Can you work these out from the model? Positions are in its coordinate system, mm. A direction names the side the tool comes from. Give positions to 0.01 mm unless a question says otherwise; leave off trailing zeros. Order: outer loops, then holes, each group sorted by start corner. A loop starts at its lowest first (then second) coordinate and runs counter-clockwise, first axis right, second up. Notation, with made-up numbers: (65.5, -12) -> (117.5, -12) arc R33 cw to (117.5, 20) -> close; hole circle Ø11 at (-12.75, -12). An arc over 180 degrees is marked (long way). Answer as CSV lines item,"result".
```python
from build123d import *

# Parameters (mm, degrees)
BOSS_EXTRUDE1_DEPTH = 5
SCALE2_SCALE        = 1.55
CUT_EXTRUDE1_DEPTH  = 12.4
BOSS_EXTRUDE3_DEPTH = 7.75
SKETCH9_W           = 20.224703408
SKETCH9_H           = 7.75
BOSS_EXTRUDE4_DEPTH = 29.5
CUT_EXTRUDE2_DEPTH  = 12.4
CHAMFER1_START      = -43
CHAMFER1_OUTLINE_W  = 8
CHAMFER1_OUTLINE_H  = 7.75
CHAMFER1_DEPTH      = 3.964353462
CHAMFER2_START      = 28.071920063
CHAMFER2_OUTLINE_W  = 8
CHAMFER2_OUTLINE_H  = 11
CHAMFER2_DEPTH      = 3.928079937
SKETCH11_R          = 0.8
CUT_EXTRUDE3_DEPTH  = 12.4
SKETCH12_R          = 0.8
CUT_EXTRUDE4_DEPTH  = 12.4
BOSS_EXTRUDE5_DEPTH = 14
SKETCH18_W          = 12
SKETCH18_H          = 3
BOSS_EXTRUDE6_DEPTH = 14
SKETCH19_R          = 2.4
BOSS_EXTRUDE7_DEPTH = 2.5
SKETCH22_W          = 3.6
SKETCH22_H          = 14
CUT_EXTRUDE5_DEPTH  = 21


with BuildPart() as part:
    # Sketch2 → Boss-Extrude1 (new body)
    with BuildSketch(Plane(origin=(0, 0, 0), x_dir=(1, 0, 0), z_dir=(0, 1, 0))):
        Polygon((-16.722011876, -36.89474357), (-23.886628792, -53.795891167), (-18.669768773, -51.685253144), (-9.373686833, -36.89474357), (-4.046151178, -17.471336145), (-4.046151178, -4.010989005), (-16.95, -4.010989005), (-14.350773449, -17.46691156), align=None)
        Polygon((-13.920870812, -6.510989005), (-6.546151178, -6.510989005), (-6.546151178, -17.13469746), (-11.686920269, -35.877181599), (-17.487790608, -45.106642876), (-14.283033348, -37.546702673), (-11.821510253, -17.379157883), align=None, mode=Mode.SUBTRACT)
    extrude(amount=BOSS_EXTRUDE1_DEPTH)


with BuildPart() as part_1:
    # Scale2: scaled about (-12.587588719, 2.5, 26.875435477)
    add(part.part.scale(SCALE2_SCALE).moved(Location((6.923173795, -1.375, -14.781489512))))

    # Sketch6 → Cut-Extrude1 (cut)
    with BuildSketch(Plane(origin=(0, 6.375, 0), x_dir=(1, 0, 0), z_dir=(0, 1, 0))):
        Polygon((-3.22336053, 6.403996086), (-3.22336053, 4.689456555), (-14.654175964, 4.689456555), align=None)
    extrude(amount=-CUT_EXTRUDE1_DEPTH, mode=Mode.SUBTRACT)

    # Sketch7 → Boss-Extrude3 (add)
    with BuildSketch(Plane(origin=(0, 6.375, 0), x_dir=(1, 0, 0), z_dir=(0, 1, 0))):
        Polygon((-19.349326204, 8.564456555), (0.65163947, 8.564456555), (0.65163947, 11.564456555), align=None)
    extrude(amount=-BOSS_EXTRUDE3_DEPTH)

    # Sketch9 → Boss-Extrude4 (add)
    with BuildSketch(Plane(origin=(-1.682081089, 0, -11.214415372), x_dir=(-0.9889374035171397, 0, 0.1483334484355372), z_dir=(-0.14833344843553717, 0, -0.9889374035171395))):
        with Locations((7.752525338, 2.5)):
            Rectangle(SKETCH9_W, SKETCH9_H)
    extrude(amount=BOSS_EXTRUDE4_DEPTH)

    # Sketch10 → Cut-Extrude2 (cut)
    with BuildSketch(Plane(origin=(0, 6.375, 0), x_dir=(1, 0, 0), z_dir=(0, 1, 0))):
        Polygon((-19.596381503, 33.807058712), (-15.888045292, 9.083623624), (-2.809641442, 11.045289485), (-6.517977653, 35.768724573), align=None)
    extrude(amount=-CUT_EXTRUDE2_DEPTH, mode=Mode.SUBTRACT)

    # Chamfer1: read off the stored shape, not the designer's step
    # Chamfer1 outline → Chamfer1 (cut)
    with BuildSketch(Plane(origin=(0, 0, 0), x_dir=(0.594396756930434, 0, -0.8041719314615392), z_dir=(0.8041719314615392, 0, 0.5943967569304341)).offset(CHAMFER1_START)):
        with Locations((16, 2.5)):
            Rectangle(CHAMFER1_OUTLINE_W, CHAMFER1_OUTLINE_H)
    extrude(amount=CHAMFER1_DEPTH, mode=Mode.SUBTRACT)

    # Chamfer2: read off the stored shape, not the designer's step
    # Chamfer2 outline → Chamfer2 (cut)
    with BuildSketch(Plane(origin=(0, 0, 0), x_dir=(0.8041719314615399, 0, 0.594396756930433), z_dir=(0.594396756930433, 0, -0.80417193146154)).offset(CHAMFER2_START)):
        with Locations((-27, -2.5)):
            Rectangle(CHAMFER2_OUTLINE_W, CHAMFER2_OUTLINE_H)
    extrude(amount=CHAMFER2_DEPTH, mode=Mode.SUBTRACT)

    # Sketch11 → Cut-Extrude3 (cut)
    with BuildSketch(Plane(origin=(0, 6.375, 0), x_dir=(1, 0, 0), z_dir=(0, 1, 0))):
        with Locations(Location((-13.316763113, 36.518532099, 0), (0, 0, 270))):
            Circle(SKETCH11_R)
    extrude(amount=-CUT_EXTRUDE3_DEPTH, mode=Mode.SUBTRACT)

    # Sketch12 → Cut-Extrude4 (cut)
    with BuildSketch(Plane(origin=(0, 6.375, 0), x_dir=(1, 0, 0), z_dir=(0, 1, 0))):
        with Locations(Location((-9.089259832, 8.333816099, 0), (0, 0, 270))):
            Circle(SKETCH12_R)
    extrude(amount=-CUT_EXTRUDE4_DEPTH, mode=Mode.SUBTRACT)

    # Sketch17 → Boss-Extrude5 (add)
    with BuildSketch(Plane(origin=(0, 6.375, 0), x_dir=(1, 0, 0), z_dir=(0, 1, 0))):
        Polygon((-17.638379984, 20.753084986), (-17.742213398, 21.445341168), (-19.418381365, 32.620333828), (-22.879662277, 32.101166759), (-21.099660896, 20.233917916), align=None)
        Polygon((-2.878696603, 35.101166759), (-6.339977515, 34.581999689), (-4.663809548, 23.407007029), (-4.559976134, 22.714750847), (-1.098695221, 23.233917916), align=None)
    extrude(amount=BOSS_EXTRUDE5_DEPTH)

    # Sketch18 → Boss-Extrude6 (add)
    with BuildSketch(Plane(origin=(-14.205964203, 0, 2.130791748), x_dir=(-0.1483334484355373, 0, -0.9889374035171397), z_dir=(0.9889374035171395, 0, -0.14833344843553728))):
        with Locations((29.139863709, 18.875)):
            Rectangle(SKETCH18_W, SKETCH18_H)
    extrude(amount=BOSS_EXTRUDE6_DEPTH)

    # Sketch19 → Boss-Extrude7 (add)
    with BuildSketch(Plane(origin=(0, 20.375, 0), x_dir=(1, 0, 0), z_dir=(0, 1, 0))):
        with Locations(Location((-11.989048632, 27.694039925, 0), (0, 0, 270))):
            Circle(SKETCH19_R)
    extrude(amount=BOSS_EXTRUDE7_DEPTH)

    # Sketch22 → Cut-Extrude5 (cut)
    with BuildSketch(Plane(origin=(-17.667245116, 0, 2.649958817), x_dir=(0.1483334484355372, 0, 0.9889374035171397), z_dir=(-0.9889374035171395, 0, 0.14833344843553717))):
        with Locations((-24.939863709, 13.375)):
            Rectangle(SKETCH22_W, SKETCH22_H)
        with Locations((-33.339863709, 13.375)):
            Rectangle(SKETCH22_W, SKETCH22_H)
    extrude(amount=-CUT_EXTRUDE5_DEPTH, mode=Mode.SUBTRACT)


solid = part_1.part
```
Item 1: Imagine slicing it at A-A, the plane y = 15.75. Please give me the cut outline in (x, z).
Numbers:
outline,"(-22.35, -28.54) -> (-18.88, -29.06) -> (-18.17, -24.31) -> (-21.63, -23.79) -> close; (-5.81, -31.02) -> (-2.34, -31.54) -> (-1.63, -26.79) -> (-5.09, -26.27) -> close"
Item 2: We'd pull the mould along X, two halves only. Please class faces 1 (the flat face through (-9.019, 2.554, -5.535)), 2 (the flat face through (-14.91, 2.45, 54.03)), 3 (the flat face through (-16, 6.375, -35)): released by +X, released by -X, zero draft, split by the parting line, or undercut.
Numbers:
face 1,"undercut"
face 2,"released by +X"
face 3,"zero draft"
Item 3: For pin 1 (6 mm diameter, centred on y = 4.5, z = 27.5, fed in from -X); pin 2 (7.5 mm diameter, centred on x = -14.5, z = -29, fed in from -Y) (3 decimals); pin 3 (2.5 mm diameter, centred on x = -13.32, z = -36.52, fed in from -Y) (3 decimals); pin 4 (1 mm diameter, centred on x = -9.09, z = -8.33, fed in from -Y), each with a flat end and sliding along its axis, tell me the tip position at first contact or that it passes through.
Numbers:
pin 1,"stops at x = -17.54"
pin 2,"stops at y = 17.375"
pin 3,"stops at y = -1.375"
pin 4,"passes through"
Item 4: For faces 4 (the flat face through (-17.363, 2.446, 1.718)), 5 (the flat face through (-13.335, 2.446, 28.005)), 6 (the flat face through (-21.756, 2.554, -36.239)), 7 (the flat face through (-26.115, 2.446, 66.989)), 8 (the cylindrical face through (-11.88, 21.61, -30.09)), which set-ups out of +Z, -Z, +X, -X, +Y, -Y let a thin tool reach every point of the face, with its end or its side?
Numbers:
face 4,"-X, +Y, -Y"
face 5,"+Y, -Y"
face 6,"-Z, -X, +Y, -Y"
face 7,"+Z, +X, +Y, -Y"
face 8,"+Y"
Item 5: Imagine slicing it at C-C, the plane y = 4.5. Please give me the cut outline in (x, z).
Numbers:
outline,"(-30.1, 68.6) -> (-19, 42.41) -> (-15.32, 12.29) -> (-19.35, -8.56) -> (-23.21, -34.28) -> (-20.26, -38.26) -> (-7.19, -40.22) -> (-3.21, -37.28) -> (0.65, -11.56) -> (0.65, 12.3) -> (-7.61, 42.41) -> (-22.01, 65.33) -> close; hole (-20.18, 55.13) -> (-15.22, 43.42) -> (-11.4, 12.16) -> (-14.65, -4.69) -> (-3.22, -6.4) -> (-3.22, 11.78) -> (-11.19, 40.83) -> close; hole (-19.6, -33.81) -> (-6.52, -35.77) -> (-2.81, -11.05) -> (-15.89, -9.08) -> close; hole circle Ø1.6 at (-13.32, -36.52); hole circle Ø1.6 at (-9.09, -8.33)"
Item 6: Please list where these lines run through material, in increasing order: line 1 along X through (y, z) = (4, 45.5); line 2 along X through (y, z) = (4, 2); line 3 along Y through (x, z) = (-18, 52.5) (3 decimals).
Numbers:
line 1,"x = -20.31 to -16.1, -14.13 to -9.55"
line 2,"x = -17.31 to -13.36, -3.22 to 0.65"
line 3,"y = -1.375 to 6.375"
Item 7: Imagine slicing it at D-D, the plane z = 57. Please give me the cut outline in (x, y) (3 decimals), then the cut area to 3 significant figures.
Numbers:
outline,"(-25.183, -1.375) -> (-16.779, -1.375) -> (-16.779, 6.375) -> (-25.183, 6.375) -> close"
area,"65.1 mm²"
Item 8: Imagine slicing it at B-B, the plane z = 34.5. Please give me the cut outline in (x, y) (3 decimals), then the cut area to 3 significant figures.
Numbers:
outline,"(-18.031, -1.375) -> (-14.127, -1.375) -> (-14.127, 6.375) -> (-18.031, 6.375) -> close; (-9.456, -1.375) -> (-5.438, -1.375) -> (-5.438, 6.375) -> (-9.456, 6.375) -> close"
area,"61.4 mm²"
